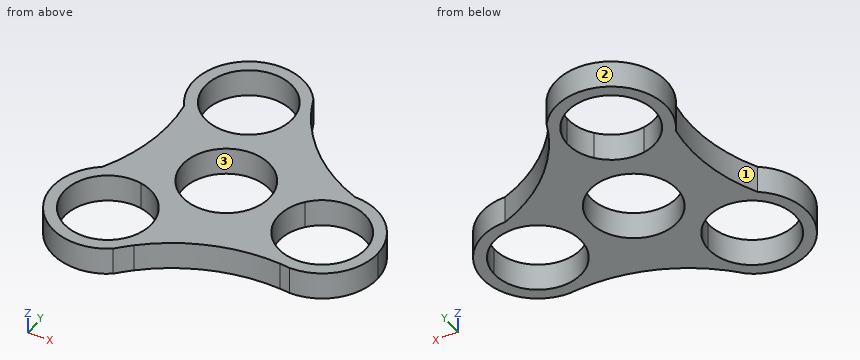
from build123d import *

# Parameters (mm, degrees)
F0_R     = 11
F1_DEPTH = 7


with BuildPart() as f1:
    # F0 (on Top) → F1 (new body)
    with BuildSketch(Plane.XY):
        with BuildLine():
            ThreePointArc((-25.5157140459, -9.3186724491), (-20.5076802891, -7.1172371315), (-15.0383400996, -7.0030554454))
            Line((-15.0383400996, -7.0030554454), (-11.7072511448, 11.7530731792))
            ThreePointArc((-11.7072511448, 11.7530731792), (-16.8027987362, 13.743579223), (-20.7465280977, 17.5348479143))
            ThreePointArc((-20.7465280977, 17.5348479143), (-20.9101748534, 3.7136476237), (-25.5157140459, -9.3186724491))
        make_face()
        with BuildLine():
            Line((-7.1451766465, -17.0378932968), (-4.3248343733, -16.0153134895))
            ThreePointArc((-4.3248343733, -16.0153134895), (-8.474173604, -10.0738468637), (-15.0383400996, -7.0030554454))
            Line((-15.0383400996, -7.0030554454), (-15.5629311457, -9.956833405))
            ThreePointArc((-15.5629311457, -9.956833405), (-10.4053717563, -12.3695980908), (-7.1451766465, -17.0378932968))
        make_face()
        with BuildLine():
            ThreePointArc((-3.4864316481, -20.78735259), (-3.6976252848, -18.364788024), (-4.3248343733, -16.0153134895))
            Line((-4.3248343733, -16.0153134895), (-7.1451766465, -17.0378932968))
            ThreePointArc((-7.1451766465, -17.0378932968), (-6.6523695055, -18.8839090024), (-6.4864316481, -20.78735259))
            ThreePointArc((-6.4864316481, -20.78735259), (-25.9172828959, -27.8528141629), (-15.5629311457, -9.956833405))
            Line((-15.5629311457, -9.956833405), (-15.0383400996, -7.0030554454))
            ThreePointArc((-15.0383400996, -7.0030554454), (-20.5076802891, -7.1172371315), (-25.5157140459, -9.3186724491))
            ThreePointArc((-25.5157140459, -9.3186724491), (-28.9551117891, -28.8166349879), (-9.4571492503, -32.256032731))
            ThreePointArc((-9.4571492503, -32.256032731), (-7.8553926266, -30.5950118305), (-6.1655412039, -29.0237012683))
            ThreePointArc((-6.1655412039, -29.0237012683), (-4.1730461617, -25.1179145502), (-3.4864316481, -20.78735259))
        make_face()
        with BuildLine():
            ThreePointArc((24.3025684766, -18.5352141326), (17.7353030809, -15.4651802248), (13.5839939697, -9.5220568343))
            Line((13.5839939697, -9.5220568343), (-4.3248343733, -16.0153134895))
            ThreePointArc((-4.3248343733, -16.0153134895), (-3.6976252848, -18.364788024), (-3.4864316481, -20.78735259))
            ThreePointArc((-3.4864316481, -20.78735259), (-4.1730461617, -25.1179145502), (-6.1655412039, -29.0237012683))
            ThreePointArc((-6.1655412039, -29.0237012683), (8.0319642762, -20.7683752456), (24.3025684766, -18.5352141326))
        make_face()
        with BuildLine():
            Line((-4.3248343733, -16.0153134895), (13.5839939697, -9.5220568343))
            ThreePointArc((13.5839939697, -9.5220568343), (12.9612940998, -2.3019261853), (16.0320855181, 4.2622403103))
            Line((16.0320855181, 4.2622403103), (1.4543461299, 16.5251122797))
            ThreePointArc((1.4543461299, 16.5251122797), (-4.4871204958, 12.375773049), (-11.7072511448, 11.7530731792))
            Line((-11.7072511448, 11.7530731792), (-15.0383400996, -7.0030554454))
            ThreePointArc((-15.0383400996, -7.0030554454), (-8.474173604, -10.0738468637), (-4.3248343733, -16.0153134895))
        make_face()
        Circle(F0_R, mode=Mode.SUBTRACT)
        with BuildLine():
            ThreePointArc((-11.7072511448, 11.7530731792), (-4.4871204958, 12.375773049), (1.4543461299, 16.5251122797))
            Line((1.4543461299, 16.5251122797), (-0.8414050971, 18.456310432))
            ThreePointArc((-0.8414050971, 18.456310432), (-5.5097003031, 15.1961153222), (-11.1826600987, 14.7068511388))
            Line((-11.1826600987, 14.7068511388), (-11.7072511448, 11.7530731792))
        make_face()
        with BuildLine():
            Line((-0.8414050971, 18.456310432), (1.4543461299, 16.5251122797))
            ThreePointArc((1.4543461299, 16.5251122797), (3.8935792851, 20.7409695987), (4.7408404036, 25.5373703238))
            ThreePointArc((4.7408404036, 25.5373703238), (4.6314684694, 27.2839246284), (4.3050615552, 29.003189787))
            ThreePointArc((4.3050615552, 29.003189787), (3.1997634843, 31.2409281113), (2.228208905, 33.5398927333))
            ThreePointArc((2.228208905, 33.5398927333), (-17.2616820059, 37.0247388251), (-20.7465280977, 17.5348479143))
            ThreePointArc((-20.7465280977, 17.5348479143), (-16.8027987362, 13.743579223), (-11.7072511448, 11.7530731792))
            Line((-11.7072511448, 11.7530731792), (-11.1826600987, 14.7068511388))
            ThreePointArc((-11.1826600987, 14.7068511388), (-16.3246211692, 33.9682215716), (1.7408404036, 25.5373703238))
            ThreePointArc((1.7408404036, 25.5373703238), (1.0751352391, 21.7687697541), (-0.8414050971, 18.456310432))
        make_face()
        with BuildLine():
            Line((1.4543461299, 16.5251122797), (16.0320855181, 4.2622403103))
            ThreePointArc((16.0320855181, 4.2622403103), (20.8367678682, 7.9419405985), (26.7455912444, 9.2499822662))
            ThreePointArc((26.7455912444, 9.2499822662), (13.7242771945, 17.0805133511), (4.3050615552, 29.003189787))
            ThreePointArc((4.3050615552, 29.003189787), (4.6314684694, 27.2839246284), (4.7408404036, 25.5373703238))
            ThreePointArc((4.7408404036, 25.5373703238), (3.8935792851, 20.7409695987), (1.4543461299, 16.5251122797))
        make_face()
        with BuildLine():
            Line((13.5839939697, -9.5220568343), (16.4043362428, -8.499477027))
            ThreePointArc((16.4043362428, -8.499477027), (15.9150720594, -2.8265172314), (18.3278367452, 2.331042158))
            Line((18.3278367452, 2.331042158), (16.0320855181, 4.2622403103))
            ThreePointArc((16.0320855181, 4.2622403103), (12.9612940998, -2.3019261853), (13.5839939697, -9.5220568343))
        make_face()
        with BuildLine():
            ThreePointArc((37.7455912444, -4.7500177338), (28.649034832, -15.5840798763), (16.4043362428, -8.499477027))
            Line((16.4043362428, -8.499477027), (13.5839939697, -9.5220568343))
            ThreePointArc((13.5839939697, -9.5220568343), (17.7353030809, -15.4651802248), (24.3025684766, -18.5352141326))
            ThreePointArc((24.3025684766, -18.5352141326), (25.525635115, -18.624927579), (26.7455912444, -18.7500177338))
            ThreePointArc((26.7455912444, -18.7500177338), (36.645086181, -14.6495126704), (40.7455912444, -4.7500177338))
            ThreePointArc((40.7455912444, -4.7500177338), (36.645086181, 5.1494772028), (26.7455912444, 9.2499822662))
            ThreePointArc((26.7455912444, 9.2499822662), (20.8367678682, 7.9419405985), (16.0320855181, 4.2622403103))
            Line((16.0320855181, 4.2622403103), (18.3278367452, 2.331042158))
            ThreePointArc((18.3278367452, 2.331042158), (30.5141918142, 5.5842771017), (37.7455912444, -4.7500177338))
        make_face()
    extrude(amount=F1_DEPTH)


solid = f1.part
Verification items for the finished model (mm, model axes). Face numbers are marked on the shaded views. Coordinates: 2 decimals unless noted, no trailing zeros. Order: outer loops, then holes, each group sorted by start corner. A loop starts at its lowest first (then second) coordinate and runs counter-clockwise, first axis right, second up. Notation, with made-up numbers: (1, 3.5) -> (16, 3.5) arc R25 ccw to (16, 18.5) -> close; hole circle Ø2 at (9.5, 77.25). An arc over 180 degrees is marked (long way). Use CSV: the item, a comma, the result in double quotes. Start each with the question number.
Q1. Depth check by flat-ended pin: P1, Ø1, axis at y = -9.5, z = 4.5, coming from the -X side; P2, Ø4, axis at x = -3, z = 1, coming from the -Y side; P3, Ø1.5, axis at x = 23.5, z = 3.5, coming from the +Y side; P4, Ø8, axis at x = 7, y = 25, coming from the -Z side. Enter the tip coordinate at first touch or a pass-through.
Q2. Section check A-A, the plane x = -24.5. Record the cut outline in (y, z), and give its area (3 significant figures).
Q3. Section check C-C, the plane y = 0. Record the cut outline in (x, z), and give its area (3 significant figures).
Q4. Section check B-B, the plane y = 27.5. Record the cut outline in (x, z), and give its area (3 significant figures).
Q5. Draft check along X on the marked faces 1, 2 and 3. Enter one of: +X half, -X half, draft (parallel to the pull), parting line (faces both ways), or undercut.
Q6. Thickness scan on line 1 along Y through (x, z) = (-15, 5); line 2 along Y through (x, z) = (-2, 4); line 3 along X through (y, z) = (32.5, 4.75). Record the ranges inside material, lowest first.
Q7. Section check D-D, the plane x = -8.5. Record the cut outline in (y, z), and give its area (3 significant figures).
Returned:
1,P1,"stops at x = -26.41"
1,P2,"stops at y = -28.03"
1,P3,"stops at y = 11"
1,P4,"stops at z = 0"
2,outline,"(-32.9, 0) -> (-29.26, 0) -> (-29.26, 7) -> (-32.9, 7) -> close; (-12.31, 0) -> (-7.36, 0) -> (-7.36, 7) -> (-12.31, 7) -> close"
2,area,"60.2 mm^2"
3,outline,"(-21.74, 0) -> (-11, 0) -> (-11, 7) -> (-21.74, 7) -> close; (11, 0) -> (16.82, 0) -> (16.82, 7) -> (11, 7) -> close; (36.67, 0) -> (39.92, 0) -> (39.92, 7) -> (36.67, 7) -> close"
3,area,"139 mm^2"
4,outline,"(-23.12, 0) -> (-20.08, 0) -> (-20.08, 7) -> (-23.12, 7) -> close; (1.56, 0) -> (5.14, 0) -> (5.14, 7) -> (1.56, 7) -> close"
4,area,"46.3 mm^2"
5,face 1,"-X half"
5,face 2,"parting line"
5,face 3,"undercut"
6,line 1,"y = -34.56 to -31.5, -10.07 to 16.15, 34.92 to 38.31"
6,line 2,"y = -25.79 to -10.82, 10.82 to 17.27, 33.8 to 37.51"
6,line 3,"x = -21.41 to -17.78, -0.74 to 2.65"
7,outline,"(-31.24, 0) -> (-27.13, 0) -> (-27.13, 7) -> (-31.24, 7) -> close; (-14.44, 0) -> (-6.98, 0) -> (-6.98, 7) -> (-14.44, 7) -> close; (6.98, 0) -> (14.56, 0) -> (14.56, 7) -> (6.98, 7) -> close; (36.51, 0) -> (39.52, 0) -> (39.52, 7) -> (36.51, 7) -> close"
7,area,"155 mm^2"
